```python
from build123d import *

# Parameters (mm, degrees)
SKETCH1_R           = 14
BOSS_EXTRUDE1_DEPTH = 17
SKETCH2_R           = 10
BOSS_EXTRUDE2_DEPTH = 45
CUT_EXTRUDE1_DEPTH  = 16


with BuildPart() as part:
    # Sketch1 → Boss-Extrude1 (new body)
    with BuildSketch(Plane.XY):
        Circle(SKETCH1_R)
    extrude(amount=-BOSS_EXTRUDE1_DEPTH)

    # Sketch2 → Boss-Extrude2 (add)
    with BuildSketch(Plane(origin=(0, 0, -17), x_dir=(-1, 0, 0), z_dir=(0, 0, -1))):
        Circle(SKETCH2_R)
    extrude(amount=BOSS_EXTRUDE2_DEPTH)

    # Sketch3 → Cut-Extrude1 (cut)
    with BuildSketch(Plane.XY):
        Polygon((5.601358059, 10.097431417), (-5.943953091, 9.899634083), (-11.54531115, -0.197797334), (-5.601358059, -10.097431417), (5.943953091, -9.899634083), (11.54531115, 0.197797334), align=None)
    extrude(amount=-CUT_EXTRUDE1_DEPTH, mode=Mode.SUBTRACT)


solid = part.part
```
The listing builds one solid part. Answer for the finished solid, in the listing's coordinates (mm). A direction names the side the tool comes from. Coordinates: 2 decimals unless noted, no trailing zeros. Order: outer loops, then holes, each group sorted by start corner. A loop starts at its lowest first (then second) coordinate and runs counter-clockwise, first axis right, second up. Notation, with made-up numbers: M -15.5,5 L 4.5,5 A18 ccw 4.5,31 Z; hole C 77,7.25 d2. An arc over 180 degrees is marked long. Answer as a JSON object with one key per item and string values. Group by question number.
1. A tool of negligible diameter and unlimited length cuts with its end or side. For faces 1 (the flat face through (-8.6, -5.1, -7.9)), 2 (the cylindrical face through (2.17, -9.76, -39.18)), 3 (the flat face through (-8.4, -6.2, 0)), from which of +Z, -Z, +X, -X, +Y, -Y can it reach the whole face along a straight path? Write none if from no direction.
2. Section C-C on y = -4.75 is taken. Write down the section's boundary in (x, z), then the cut area to 3 significant figures.
3. Straight lines are drawn through the part: line 1 (X direction, y = -0.25, z = -41.5); line 2 (Z direction, x = -12, y = -2.5); line 3 (Y direction, x = -6.5, z = -13). For each, find the intervals that lie inside material, in ascending order.
4. Section D-D on z = -22 is taken. Write down the section's boundary in (x, y).
5. Section A-A on z = -10 is taken. Write down the section's boundary in (x, y).
6. Flat-ended cylindrical pins translate along their axes: P1, Ø6, axis at x = -1, y = -1.5, coming from the +Z side; P2, Ø10, axis at y = 3, z = -48.5, coming from the +X side; P3, Ø5, axis at x = 8.5, z = -53, coming from the -Y side. Find the tip coordinate at first contact, or state that the pin passes through.
7. Determine the mould class of faces 4 (the flat face through (8.6, 5.1, -7.9)), 5 (the cylindrical face through (12.932, -5.362, -8.381)), 6 (the flat face through (-3, 10, -17)) for opening direction Y: released by +Y, released by -Y, zero draft, split by the parting line, or undercut.
8. Section B-B on x = 1.5 is taken. Write down the section's boundary in (y, z).
Values follow:
{
 "1": {"face 1": "+Z", "face 2": "-Z", "face 3": "+Z, +X, -X, +Y, -Y"},
 "2": {"outline": "M -13.17,-17 L -8.8,-17 L -8.8,-62 L 8.8,-62 L 8.8,-17 L 13.17,-17 L 13.17,0 L 8.8,0 L 8.8,-16 L -8.81,-16 L -8.81,0 L -13.17,0 Z", "area": "958 mm2"},
 "3": {"line 1": "-10 to 10", "line 2": "-17 to 0", "line 3": "-12.4 to -8.6, 8.9 to 12.4"},
 "4": {"outline": "C 0,0 d20"},
 "5": {"outline": "C 0,0 d28; hole M -11.55,-0.2 L -5.6,-10.1 L 5.94,-9.9 L 11.55,0.2 L 5.6,10.1 L -5.94,9.9 Z"},
 "6": {"P1": "z = -16", "P2": "x = 10", "P3": "y = -8"},
 "7": {"face 4": "undercut", "face 5": "split by the parting line", "face 6": "zero draft"},
 "8": {"outline": "M -13.92,-17 L -9.89,-17 L -9.89,-62 L 9.89,-62 L 9.89,-17 L 13.92,-17 L 13.92,0 L 10.03,0 L 10.03,-16 L -9.98,-16 L -9.98,0 L -13.92,0 Z"}
}
